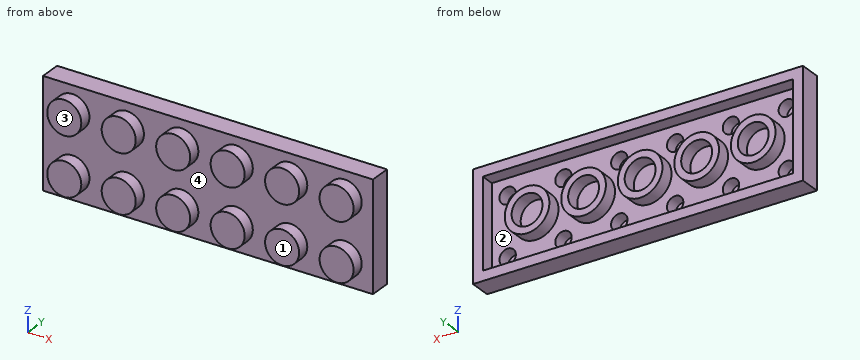
```python
from build123d import *

# Parameters (mm, degrees)
F0_W      = 47.86
F0_H      = 15.8
F1_DEPTH  = 3.09
F2_R      = 2.47
F3_DEPTH  = 1.79
F4_W      = 45.02
F4_H      = 12.96
F5_DEPTH  = 2
F6_R      = 3.24
F7_DEPTH  = 2
F8_R      = 2.24
F9_DEPTH  = 2.2
F10_R     = 1.19
F11_DEPTH = 1.9


with BuildPart() as f1:
    # F0 (on Front) → F1 (new body)
    with BuildSketch(Plane.XZ):
        with Locations((23.93, 7.9)):
            Rectangle(F0_W, F0_H)
    extrude(amount=F1_DEPTH)

    # F2 (on face) → F3 (join)
    with BuildSketch(Plane.XZ.offset(3.09)):
        with Locations((4.263951, 12.12003)):
            Circle(F2_R)
        with Locations((12.163951, 12.12003)):
            Circle(F2_R)
        with Locations((20.063951, 12.12003)):
            Circle(F2_R)
        with Locations((27.963951, 12.12003)):
            Circle(F2_R)
        with Locations((35.863951, 12.12003)):
            Circle(F2_R)
        with Locations((43.763951, 12.12003)):
            Circle(F2_R)
        with Locations((4.263951, 3.674378)):
            Circle(F2_R)
        with Locations((12.163951, 3.674378)):
            Circle(F2_R)
        with Locations((20.063951, 3.674378)):
            Circle(F2_R)
        with Locations((27.963951, 3.674378)):
            Circle(F2_R)
        with Locations((35.863951, 3.674378)):
            Circle(F2_R)
        with Locations((43.763951, 3.674378)):
            Circle(F2_R)
    extrude(amount=F3_DEPTH)

    # F4 (on face) → F5 (cut)
    with BuildSketch(Plane(origin=(0, 0, 0), x_dir=(-1, 0, 0), z_dir=(0, 1, 0))):
        with Locations((-23.93, 7.9)):
            Rectangle(F4_W, F4_H)
    extrude(amount=-F5_DEPTH, mode=Mode.SUBTRACT)

    # F6 (on face) → F7 (join, through all)
    with BuildSketch(Plane(origin=(0, -2, 0), x_dir=(-1, 0, 0), z_dir=(0, 1, 0))):
        with Locations((-40.02, 7.9)):
            Circle(F6_R)
        with Locations((-31.82, 7.9)):
            Circle(F6_R)
        with Locations((-23.62, 7.9)):
            Circle(F6_R)
        with Locations((-15.42, 7.9)):
            Circle(F6_R)
        with Locations((-7.22, 7.9)):
            Circle(F6_R)
    extrude(amount=F7_DEPTH)

    # F8 (on face) → F9 (cut)
    with BuildSketch(Plane(origin=(0, -2, 0), x_dir=(-1, 0, 0), z_dir=(0, 1, 0))):
        with Locations((-40.02, 7.9)):
            Circle(F8_R)
        with Locations((-31.82, 7.9)):
            Circle(F8_R)
        with Locations((-23.62, 7.9)):
            Circle(F8_R)
        with Locations((-15.42, 7.9)):
            Circle(F8_R)
        with Locations((-7.22, 7.9)):
            Circle(F8_R)
    extrude(amount=F9_DEPTH, mode=Mode.SUBTRACT)

    # F10 (on face) → F11 (cut)
    with BuildSketch(Plane(origin=(0, -2, 0), x_dir=(-1, 0, 0), z_dir=(0, 1, 0))):
        with Locations((-44.157173, 11.981434)):
            Circle(F10_R)
        with Locations((-44.157173, 3.501521)):
            Circle(F10_R)
        with Locations((-36.057173, 11.981434)):
            Circle(F10_R)
        with Locations((-36.057173, 3.501521)):
            Circle(F10_R)
        with Locations((-27.957173, 11.981434)):
            Circle(F10_R)
        with Locations((-27.957173, 3.501521)):
            Circle(F10_R)
        with Locations((-19.857173, 11.981434)):
            Circle(F10_R)
        with Locations((-19.857173, 3.501521)):
            Circle(F10_R)
        with Locations((-11.757173, 11.981434)):
            Circle(F10_R)
        with Locations((-11.757173, 3.501521)):
            Circle(F10_R)
        with Locations((-3.657173, 11.981434)):
            Circle(F10_R)
        with Locations((-3.657173, 3.501521)):
            Circle(F10_R)
    extrude(amount=-F11_DEPTH, mode=Mode.SUBTRACT)


solid = f1.part
```
Here's how the part is built. I have some questions about the finished solid (model axes, mm). Face numbers are marked on the shaded views. A direction names the side the tool comes from. Give positions to 0.01 mm unless a question says otherwise; leave off trailing zeros. Loops run counter-clockwise (first coordinate to the right, second up) from the corner with the lowest first, then second, coordinate; pieces in that order, holes last. Notation, with made-up numbers: M 18.5,88.25 L 74.5,88.25 A35 ccw 74.5,122.25 Z; hole C 17,-29.5 d11. An arc over 180 degrees is marked long. Put each result on its own line as item: value. Start each with the question number.
(1) Will these pins go through, and if not, where does the flat tip stop? pin 1 Ø3 at (x, z) = (36.06, 3.5) entering from +Y; pin 2 Ø6 at (x, z) = (31.82, 7.9) entering from -Y.
(2) If we mould it in two halves opening along Z, with no side actions, what happens to the marked faces 3 and 4? For each: +Z half, -Z half, draft (parallel to the pull), parting line (faces both ways), or undercut.
(3) I want a section at B-B on x = 14. Please give me the cut outline in (y, z), then the cut area to 3 significant figures.
(4) For the marked faces 1 and 2, which set-ups out of +Z, -Z, +X, -X, +Y, -Y let a thin tool reach every point of the face, with its end or its side?
(5) I want a section at A-A on x = 31.82. Please give me the cut outline in (y, z).
(6) I need wall thicknesses on line 1 along Z through (x, y) = (7.22, -0.65); line 2 along X through (y, z) = (-0.25, 11.75); line 3 along Z through (x, y) = (35.5, -1.9). Which ranges of each line are inside material? Lowest first, please. Write a range as [from, to].
Answer block:
1. pin 1: y = -2
1. pin 2: y = -3.09
2. face 3: draft
2. face 4: undercut
3. outline: M -4.88,2.02 L -3.09,2.02 L -3.09,0 L 0,0 L 0,1.42 L -2,1.42 L -2,4.99 L 0,4.99 L 0,6.17 L -2,6.17 L -2,9.63 L 0,9.63 L 0,10.81 L -2,10.81 L -2,14.38 L 0,14.38 L 0,15.8 L -3.09,15.8 L -3.09,13.77 L -4.88,13.77 L -4.88,10.47 L -3.09,10.47 L -3.09,5.33 L -4.88,5.33 Z
3. area: 39.5 mm^2
4. face 1: +Z, -Z, +X, -X, -Y
4. face 2: +Y
5. outline: M -3.09,0 L 0,0 L 0,1.42 L -2,1.42 L -2,4.66 L 0,4.66 L 0,5.66 L -2,5.66 L -2,10.14 L 0,10.14 L 0,11.14 L -2,11.14 L -2,14.38 L 0,14.38 L 0,15.8 L -3.09,15.8 Z
6. line 1: [0, 1.42], [4.66, 5.66], [10.14, 11.14], [14.38, 15.8]
6. line 2: [0, 1.42], [46.44, 47.86]
6. line 3: [0, 1.42], [14.38, 15.8]
